Geometry: final body of the model. Coordinates: model frame, mm. A direction names the side the tool comes from. Give positions to 0.01 mm unless a question says otherwise; leave off trailing zeros. Write each loop counter-clockwise with the first axis right and the second up, starting at its lowest first coordinate (ties: lowest second). Pieces come first, ordered by that corner, then holes. Notation, with made-up numbers: M 43.25,6.25 L 91.25,6.25 A16 ccw 91.25,12.25 Z; hole C 29.25,-23.5 d9. An arc over 180 degrees is marked long. Use a Markdown table: item, result. Add a question column.
1) Section A-A on y = 0. Return the cut outline in (x, z).
2) Line query: line 1 (X direction, y = 12, z = 25.5); line 2 (Z direction, x = 0, y = -15.5); line 3 (Z direction, x = 11, y = 8). Output: solid intervals per line, ascending.
3) Draft query along Y for faces 1 (the flat face through (-9, 5, 35.4)), 2 (the flat face through (-9, -11, 0)), 3 (the flat face through (-25.446, -19.067, 28.173)), 4 (the flat face through (-37.966, -57.903, 15.117)). Return one class per face: +Y half, -Y half, draft (parallel to the pull), parting line (faces both ways), or undercut.
4) Section B-B on x = 0. Return the cut outline in (y, z), then the cut area to 3 significant figures.
5) Set-up query: faces 5 (the flat face through (0, 11, 35.4)), 6 (the cylindrical face through (5.723, -51.416, -8.631)), 7 (the flat face through (9, -5, 8.6)), 8 (the flat face through (-10.1, 4.1, 22.2)). Return all of +Z, -Z, +X, -X, +Y, -Y with unobstructed straight access to the full face (end or side cutting, diameter ignored); none if empty.
6) Pin query (flat end, axial travel): pin 1 (8 mm diameter, centred on x = -22, y = -83.5, fed in from +Z); pin 2 (5 mm diameter, centred on x = 4, y = -69.5, fed in from -Z); pin 3 (2.5 mm diameter, centred on x = 0.5, y = -11, fed in from +Z). Return the tip coordinate at first contact, or that it passes through.
```python
from build123d import *

# Parameters (mm, degrees)
CYLINDER002_R         = 20
CYLINDER002_DEPTH     = 10
PAD_DEPTH             = 100
CLONE_PLACEMENT_ANGLE = 18
SKETCH010_R           = 6
PAD008_DEPTH          = 3
SKETCH011_R           = 6
PAD009_DEPTH          = 10
PAD010_DEPTH          = 25
PAD010_DEPTH_BACK     = 1
CYLINDER_R            = 19
CYLINDER_DEPTH        = 57
SKETCH006_R           = 14
POCKET001_DEPTH       = 20.9027
POCKET001_DEPTH_BACK  = 57.001
SKETCH001_W           = 7.25
SKETCH001_H           = 26.8
PAD001_DEPTH          = 1.5
POLARPATTERN_COUNT    = 6


with BuildPart() as cylinder002:
    # Cylinder002 → Cylinder002 (new body)
    with BuildSketch(Plane.XY.offset(56)):
        Circle(CYLINDER002_R)
    extrude(amount=CYLINDER002_DEPTH)


with BuildPart() as cut:
    # Sketch → Pad (new body)
    with BuildSketch(Plane.XZ):
        with BuildLine():
            Line((-15.852902, 39.699504), (-8.796326, 7.096149))
            ThreePointArc((-8.796326, 7.096149), (0, 0), (8.796326, 7.096149))
            Line((8.796326, 7.096149), (15.852902, 39.699504))
            ThreePointArc((15.852902, 39.699504), (15.463392, 43.660617), (12.837838, 46.652038))
            ThreePointArc((12.837838, 46.652038), (0, 50.2), (-12.837838, 46.652038))
            ThreePointArc((-12.837838, 46.652038), (-15.463392, 43.660617), (-15.852902, 39.699504))
        make_face()
    extrude(amount=PAD_DEPTH)


with BuildPart() as cut_1:
    # Body placement: moved
    add(cut.part.moved(Location((100, 0, 0))))


with BuildPart() as cut_2:
    # Clone placement: moved
    add(cut_1.part.moved(Location((-100, 3, 10))).rotate(Axis((-100, 3, 10), (1, 0, 0)), CLONE_PLACEMENT_ANGLE))

    # Sketch010 (on Face3 of Clone) → Pad008 (new body)
    with BuildSketch(Plane(origin=(6.93556, 3.463869, 8.572357), x_dir=(0, 0.951057, 0.309017), z_dir=(0.97737, 0.065369, -0.201186))):
        with Locations((-54.5, 31)):
            Circle(SKETCH010_R)
    extrude(amount=PAD008_DEPTH)

    # Sketch011 → Pad009 (join)
    with BuildSketch(Plane(origin=(0, 0, 6), x_dir=(1, 0, 0), z_dir=(0, -0.309017, 0.951057))):
        with Locations((0, -55.223284)):
            Circle(SKETCH011_R)
    extrude(amount=PAD009_DEPTH)

    # Sketch012 (on Face1 of Pad009) → Pad010 (join, two sides)
    with BuildSketch(Plane(origin=(-6.93556, 3.463869, 8.572357), x_dir=(0, -0.951057, -0.309017), z_dir=(-0.97737, 0.065369, -0.201186))) as pad010_sk:
        with BuildLine():
            Line((16.544459, 44), (99.9, 44))
            Line((99.9, 44), (99.9, 18))
            Line((99.9, 18), (23.31369, 18))
            ThreePointArc((18.708854, 21.0518), (20.551535, 18.832207), (23.31369, 18))
            Line((18.708854, 21.0518), (11.939623, 37.0518))
            ThreePointArc((16.544459, 44), (12.376666, 41.762155), (11.939623, 37.0518))
        make_face()
    extrude(amount=PAD010_DEPTH)
    extrude(pad010_sk.sketch, amount=-PAD010_DEPTH_BACK)

    # Cut: cut Cylinder002
    add(cylinder002.part, mode=Mode.SUBTRACT)


with BuildPart() as obj1:
    # Cylinder → Cylinder (new body)
    with BuildSketch(Plane.XY):
        Circle(CYLINDER_R)
    extrude(amount=CYLINDER_DEPTH)

    # Fusion: union Cut
    add(cut_2.part)

    # Sketch006 → Pocket001 (cut, two sides)
    with BuildSketch(Plane.XY) as pocket001_sk:
        Circle(SKETCH006_R)
    extrude(amount=-POCKET001_DEPTH, mode=Mode.SUBTRACT)
    extrude(pocket001_sk.sketch, amount=POCKET001_DEPTH_BACK, mode=Mode.SUBTRACT)

    # Sketch001 → Pad001 (join, symmetric)
    with BuildSketch(Plane.YZ):
        with Locations((11.375, 22)):
            Rectangle(SKETCH001_W, SKETCH001_H)
    pad001 = extrude(amount=PAD001_DEPTH, both=True)

    # PolarPattern: Pad001 ×6 about axis
    polarpattern_axis = Axis((0, 0, 0), (0, 0, 1))
    for i in range(1, POLARPATTERN_COUNT):
        add(pad001.rotate(polarpattern_axis, i * 360 / POLARPATTERN_COUNT))


solid = obj1.part
```
Found:
| question | item | result |
|---|---|---|
| 1 | outline | M -19,0 L -14,0 L -14,57 L -19,57 Z; M 14,0 L 19,0 L 19,57 L 14,57 Z |
| 2 | line 1 | -14.73 to -7.21, -1.5 to 1.5, 7.21 to 14.73 |
| 2 | line 2 | 0 to 57 |
| 2 | line 3 | 8.6 to 35.4 |
| 3 | face 1 | undercut |
| 3 | face 2 | draft |
| 3 | face 3 | undercut |
| 3 | face 4 | +Y half |
| 4 | outline | M -107.62,26.84 L -92.11,-20.9 L -59.12,-10.18 L -58.23,-12.92 L -46.81,-9.21 L -47.7,-6.47 L -19,2.85 L -19,0 L -14,0 L -14,8.6 L -7.75,8.6 L -7.75,35.4 L -14,35.4 L -14,57 L -19,57 L -19,55.64 Z; M 7.75,8.6 L 14,8.6 L 14,0 L 19,0 L 19,57 L 14,57 L 14,35.4 L 7.75,35.4 Z |
| 4 | area | 5,210 mm² |
| 5 | face 5 | +Z |
| 5 | face 6 | none |
| 5 | face 7 | -Z |
| 5 | face 8 | +Z, -Z |
| 6 | pin 1 | z = 25.81 |
| 6 | pin 2 | z = -13.84 |
| 6 | pin 3 | z = 35.4 |
